Geometry check sheet. Reference: the model listing, model coordinates, mm. Round coordinates to 2 decimals unless told otherwise and drop trailing zeros. Write each loop counter-clockwise with the first axis right and the second up, starting at its lowest first coordinate (ties: lowest second). Pieces come first, ordered by that corner, then holes.
Item 1: Scan lines: probe 1 along X at (y, z) = (6, -140); probe 2 along Z at (x, y) = (1460, 4.5); probe 3 along X at (y, z) = (11, -76.5). Record each from-to range of solid material in increasing order.
Item 2: Cross-section at B-B (y = 3). Enter the section's corners in (x, z), then the cut area to 3 significant figures.
Item 3: Cross-section at C-C (x = 1460). Enter the section's corners in (y, z), then the cut area to 3 significant figures.
Item 4: Cross-section at A-A (z = 20). Enter the section's corners in (x, y), then the cut area to 3 significant figures.
Item 5: Depth check by flat-ended pin: P1, Ø11, axis at y = 14.5, z = -73, coming from the +X side; P2, Ø12, axis at x = 118.5, z = 21, coming from the +Y side; P3, Ø20.5, axis at x = 1460, z = -140, coming from the -Y side; P4, Ø10, axis at y = 6, z = -80.5, coming from the -X side. Enter the tip coordinate at first touch or a pass-through.
Item 6: Cross-section at D-D (z = -64.5). Enter the section's corners in (x, y).
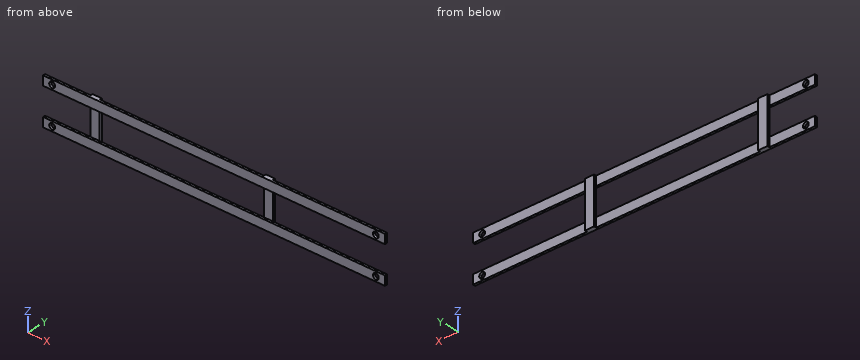
from build123d import *

# Parameters (mm, degrees)
SKETCH1_W           = 1200
SKETCH1_H           = 40
BOSS_EXTRUDE1_DEPTH = 10
SKETCH2_W           = 40
SKETCH2_H           = 200
BOSS_EXTRUDE2_DEPTH = 10
SKETCH3_W           = 1200
SKETCH3_H           = 40
BOSS_EXTRUDE3_DEPTH = 10
SKETCH5_W           = 300
SKETCH5_H           = 40
BOSS_EXTRUDE4_DEPTH = 10
SKETCH4_R           = 12.7
CUT_EXTRUDE1_DEPTH  = 10


with BuildPart() as part:
    # Sketch1 → Boss-Extrude1 (new body)
    with BuildSketch(Plane(origin=(0, 0, 0), x_dir=(1, 0, 0), z_dir=(0, 1, 0))):
        with Locations((600, -20)):
            Rectangle(SKETCH1_W, SKETCH1_H)
    extrude(amount=BOSS_EXTRUDE1_DEPTH)

    # Sketch2 → Boss-Extrude2 (add)
    with BuildSketch(Plane(origin=(0, 10, 0), x_dir=(1, 0, 0), z_dir=(0, 1, 0))):
        with Locations((220, 60)):
            Rectangle(SKETCH2_W, SKETCH2_H)
        with Locations((980, 60)):
            Rectangle(SKETCH2_W, SKETCH2_H)
    extrude(amount=BOSS_EXTRUDE2_DEPTH)

    # Sketch3 → Boss-Extrude3 (add)
    with BuildSketch(Plane.XZ.offset(-10)):
        with Locations((600, -140)):
            Rectangle(SKETCH3_W, SKETCH3_H)
    extrude(amount=BOSS_EXTRUDE3_DEPTH)

    # Sketch5 → Boss-Extrude4 (add)
    with BuildSketch(Plane(origin=(0, 10, 0), x_dir=(1, 0, 0), z_dir=(0, 1, 0))):
        with Locations((1350, 140)):
            Rectangle(SKETCH5_W, SKETCH5_H)
        with Locations((1350, -20)):
            Rectangle(SKETCH5_W, SKETCH5_H)
    extrude(amount=-BOSS_EXTRUDE4_DEPTH)

    # Sketch4 → Cut-Extrude1 (cut)
    with BuildSketch(Plane.XZ):
        with Locations(Location((1460, 20, 0), (0, 0, 270))):
            Circle(SKETCH4_R)
        with Locations(Location((40, 20, 0), (0, 0, 270))):
            Circle(SKETCH4_R)
        with Locations(Location((40, -140, 0), (0, 0, 270))):
            Circle(SKETCH4_R)
        with Locations(Location((1460, -140, 0), (0, 0, 270))):
            Circle(SKETCH4_R)
    extrude(amount=-CUT_EXTRUDE1_DEPTH, mode=Mode.SUBTRACT)


solid = part.part
Resolved:
1. probe 1: x = 0 to 27.3, 52.7 to 1447.3, 1472.7 to 1500
1. probe 2: z = -160 to -152.7, -127.3 to -120, 0 to 7.3, 32.7 to 40
1. probe 3: x = 200 to 240, 960 to 1000
2. outline: (0, -160) - (1500, -160) - (1500, -120) - (0, -120) - close; (0, 0) - (1500, 0) - (1500, 40) - (0, 40) - close; hole circle Ø25.4 at (40, -140); hole circle Ø25.4 at (40, 20); hole circle Ø25.4 at (1460, -140); hole circle Ø25.4 at (1460, 20)
2. area: 118,000 mm2
3. outline: (0, -160) - (10, -160) - (10, -152.7) - (0, -152.7) - close; (0, -127.3) - (10, -127.3) - (10, -120) - (0, -120) - close; (0, 0) - (10, 0) - (10, 7.3) - (0, 7.3) - close; (0, 32.7) - (10, 32.7) - (10, 40) - (0, 40) - close
3. area: 292 mm2
4. outline: (0, 0) - (27.3, 0) - (27.3, 10) - (0, 10) - close; (52.7, 0) - (1447.3, 0) - (1447.3, 10) - (1000, 10) - (1000, 20) - (960, 20) - (960, 10) - (240, 10) - (240, 20) - (200, 20) - (200, 10) - (52.7, 10) - close; (1472.7, 0) - (1500, 0) - (1500, 10) - (1472.7, 10) - close
4. area: 15,300 mm2
5. P1: stops at x = 1000
5. P2: stops at y = 10
5. P3: passes through
5. P4: stops at x = 200
6. outline: (200, 10) - (240, 10) - (240, 20) - (200, 20) - close; (960, 10) - (1000, 10) - (1000, 20) - (960, 20) - close
